```python
from build123d import *

# Parameters (mm, degrees)
F0_R     = 31.5
F1_DEPTH = 200
F2_R     = 49.4625151614
F2_R_2   = 15.5
F3_DEPTH = 170
F4_R     = 5
F5_R     = 19.4675976679
F6_DEPTH = 30
F6_TAPER = 3
F7_R     = 10
F8_DEPTH = 25


with BuildPart() as f1:
    # F0 (on Front) → F1 (new body)
    with BuildSketch(Plane.XZ):
        Circle(F0_R)
    extrude(amount=F1_DEPTH)

    # F2 (on face) → F3 (cut)
    with BuildSketch(Plane.XZ.offset(200)):
        Circle(F2_R)
        Circle(F2_R_2, mode=Mode.SUBTRACT)
    extrude(amount=-F3_DEPTH, mode=Mode.SUBTRACT)

    # F4
    f4_edges = [f1.edges().sort_by_distance(p)[0] for p in [
        (-15.5, -30, 0),
    ]]
    fillet(f4_edges, radius=F4_R)

    # F5 (on face) → F6 (join)
    with BuildSketch(Plane(origin=(0, 0, 0), x_dir=(-1, 0, 0), z_dir=(0, 1, 0))):
        Circle(F5_R)
    extrude(amount=F6_DEPTH, taper=F6_TAPER)

    # F7 (on face) → F8 (cut)
    with BuildSketch(Plane.XZ.offset(200)):
        Circle(F7_R)
    extrude(amount=-F8_DEPTH, mode=Mode.SUBTRACT)


solid = f1.part
```
The listing builds one solid part. Answer for the finished solid, in the listing's coordinates (mm). A direction names the side the tool comes from. Coordinates: 2 decimals unless noted, no trailing zeros. Write each loop counter-clockwise with the first axis right and the second up, starting at its lowest first coordinate (ties: lowest second). Pieces come first, ordered by that corner, then holes. Notation, with made-up numbers: (3.25, 17) - (57.25, 17) arc R33 ccw to (57.25, 47) - close; hole circle Ø11 at (51, 84). An arc over 180 degrees is marked (long way). One line per item, written item: value.
1) For a pull along Z with two mould halves and no side action, classify faces 4 (the cylindrical face through (-2.17, -187.68, -9.76)), 5 (the flat face through (21, -30, 0)), 6 (the cylindrical face through (-2.018, -118.655, 15.368)) as pulls with the +Z half, pulls with the -Z half, needs draft (parallel to the pull), parting line crosses it, or undercut.
Geometry check:
face 4: undercut
face 5: needs draft
face 6: parting line crosses it
2) Find section D-D (x = 26). Give the vertices of the cut face in (y, z).
Geometry check:
outline: (-30, -17.78) - (0, -17.78) - (0, 17.78) - (-30, 17.78) - close
3) Find section A-A (x = 0). Give the vertices of the cut face in (y, z), and give its area (3 significant figures).
Geometry check:
outline: (-200, -15.5) - (-35, -15.5) arc R5 cw to (-30, -20.5) - (-30, -31.5) - (0, -31.5) - (0, -19.47) - (30, -17.9) - (30, 17.9) - (0, 19.47) - (0, 31.5) - (-30, 31.5) - (-30, 20.5) arc R5 cw to (-35, 15.5) - (-200, 15.5) - (-200, 10) - (-175, 10) - (-175, -10) - (-200, -10) - close
area: 7,790 mm2
4) A tool of negligible diameter and unlimited length cuts with its end or side. For faces 1 (the flat face through (14, 0, 14)), 2 (the cylindrical face through (-4.101, -14.79, 31.232)), 3 (the flat face through (0, -175, 0)), from which of +Z, -Z, +X, -X, +Y, -Y can it reach the whole face along a straight path? Write none if from no direction.
Geometry check:
face 1: +Y
face 2: +Y, -Y
face 3: -Y
5) Find section B-B (y = -147). Give the vertices of the cut face in (x, z), and give its area (3 significant figures).
Geometry check:
outline: circle Ø31 at (0, 0)
area: 755 mm2
6) Find section C-C (y = -16.5). Give the vertices of the cut face in (x, z).
Geometry check:
outline: circle Ø63 at (0, 0)
7) Consider line 1 along Z through (x, y) = (0, -183); line 2 along Y through (x, z) = (11, 28); line 3 along X through (y, z) = (-179.5, -0.5). Determine where each line is inside the solid, lowest interval first. Write a range as from..to.
Geometry check:
line 1: z = -15.5..-10, 10..15.5
line 2: y = -30..0
line 3: x = -15.49..-9.99, 9.99..15.49
8) Each of these flat-tipped pins is pushed along its axis until it touches: pin 1 Ø1 at (x, y) = (9, -62.5) entering from +Z; pin 2 Ø12 at (x, y) = (7, -20.5) entering from -Z; pin 3 Ø12 at (y, z) = (-53.5, 22.5) entering from -X; pin 4 Ø6 at (x, z) = (14, -23.5) entering from -Y. Where does it stop, or does it pass through?
Geometry check:
pin 1: stops at z = 12.96
pin 2: stops at z = -31.48
pin 3: passes through
pin 4: stops at y = -30
